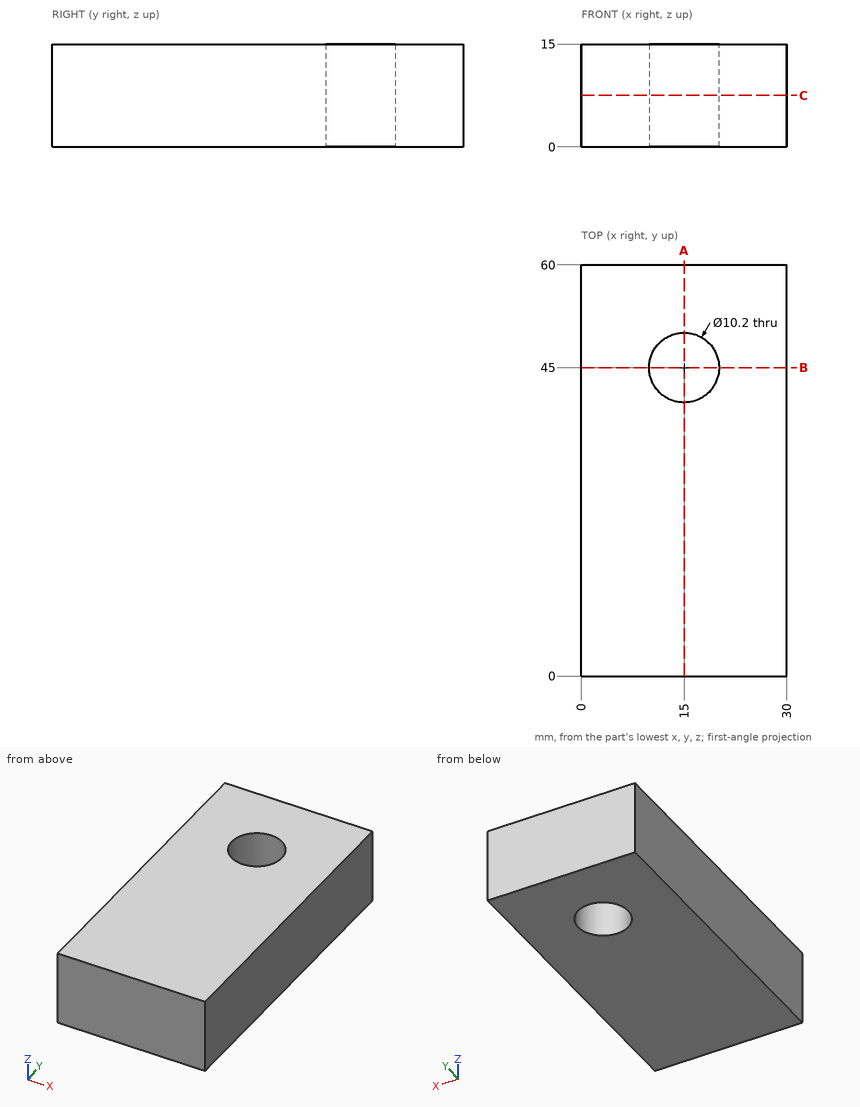
Source: three-view drawing plus pictorial views. Frame: mm from the lowest corner of the part. Give positions to 0.01 mm unless a question says otherwise; leave off trailing zeros. Order: outer loops, then holes, each group sorted by start corner. A loop starts at its lowest first (then second) coordinate and runs counter-clockwise, first axis right, second up. Notation, with made-up numbers: (31, 29.25) -> (42, 29.25) arc R14 ccw to (42, 43.25) -> close; hole circle Ø4 at (-8.75, -9.75). An arc over 180 degrees is marked (long way). Use a Markdown table: item, result.
Q1. First-contact query: P1, Ø1, axis at x = 13, y = 41.5, coming from the -Z side (3 decimals); P2, Ø5, axis at y = 31.5, z = 7, coming from the -X side. Flat tips, straight axial feed; report the tip coordinate or a pass-through.
A:
| item | result |
|---|---|
| P1 | through |
| P2 | x = 0 |
Q2. Section B-B (y = 45). Return the cut outline in (x, z), and give its area (3 significant figures).
A:
| item | result |
|---|---|
| outline | (0, 0) -> (9.9, 0) -> (9.9, 15) -> (0, 15) -> close; (20.1, 0) -> (30, 0) -> (30, 15) -> (20.1, 15) -> close |
| area | 297 mm^2 |
Q3. Section A-A (x = 15). Return the cut outline in (y, z), and give its area (3 significant figures).
A:
| item | result |
|---|---|
| outline | (0, 0) -> (39.9, 0) -> (39.9, 15) -> (0, 15) -> close; (50.1, 0) -> (60, 0) -> (60, 15) -> (50.1, 15) -> close |
| area | 747 mm^2 |
Q4. Section C-C (z = 7.5). Return the cut outline in (x, y).
A:
| item | result |
|---|---|
| outline | (0, 0) -> (30, 0) -> (30, 60) -> (0, 60) -> close; hole circle Ø10.2 at (15, 45) |
Q5. Material intervals for line 1 (X direction, y = 45, z = 3); line 2 (Y direction, x = 15, z = 11); line 3 (X direction, y = 44, z = 12.75), sorted ascending. Write a range as [from, to].
A:
| item | result |
|---|---|
| line 1 | [0, 9.9], [20.1, 30] |
| line 2 | [0, 39.9], [50.1, 60] |
| line 3 | [0, 10], [20, 30] |
